```python
from build123d import *

# Parameters (mm, degrees)
SKETCH_1_R          = 9
EXTRUDE_1_DEPTH     = 8
CUT_EXTRUDE_1_DEPTH = 16.033296378
EXTRUDE_START       = -8
SKETCH_7_R          = 23
SKETCH_7_R_2        = 9
EXTRUDE_2_DEPTH     = 8
SKETCH_8_R          = 29
SKETCH_8_R_2        = 23
EXTRUDE_3_DEPTH     = 0.5
EXTRUDE_START_2     = -0.5
SKETCH_9_R          = 29
SKETCH_9_R_2        = 23
EXTRUDE_4_DEPTH     = 0.5
SKETCH_10_R         = 1.25977889
CUT_EXTRUDE_2_DEPTH = 25


with BuildPart() as part:
    # 草圖1 → 填料-伸長1 (new body)
    with BuildSketch(Plane(origin=(0, 0, 0), x_dir=(1, 0, 0), z_dir=(0, 1, 0))):
        with Locations(Location((0, 0, 0), (0, 0, 270))):
            Circle(SKETCH_1_R)
    extrude(amount=-EXTRUDE_1_DEPTH)

    # 草圖2 → 除料-伸長1 (cut, through all)
    with BuildSketch(Plane(origin=(0, -8, 0), x_dir=(-1, 0, 0), z_dir=(0, -1, 0))):
        with BuildLine():
            Line((-0.93, 1.264911064), (-0.93, -1.264911064))
            ThreePointArc((-0.93, -1.264911064), (0.708801806, -1.400892573), (1.57, 0))
            ThreePointArc((1.57, 0), (0.708801806, 1.400892573), (-0.93, 1.264911064))
        make_face()
    extrude(amount=-CUT_EXTRUDE_1_DEPTH, mode=Mode.SUBTRACT)

    # 草圖7 → 填料-伸長2 (add)
    with BuildSketch(Plane(origin=(0, -8, 0), x_dir=(-1, 0, 0), z_dir=(0, -1, 0)).offset(EXTRUDE_START)):
        with Locations(Location((0, 0, 0), (0, 0, 90))):
            Circle(SKETCH_7_R)
        Circle(SKETCH_7_R_2, mode=Mode.SUBTRACT)
    extrude(amount=EXTRUDE_2_DEPTH)

    # 草圖8 → 填料-伸長3 (add)
    with BuildSketch(Plane(origin=(0, 0, 0), x_dir=(1, 0, 0), z_dir=(0, 1, 0))):
        with Locations(Location((0, 0, 0), (0, 0, 270))):
            Circle(SKETCH_8_R)
        with Locations(Location((0, 0, 0), (0, 0, 90))):
            Circle(SKETCH_8_R_2, mode=Mode.SUBTRACT)
    extrude(amount=-EXTRUDE_3_DEPTH)

    # 草圖9 → 填料-伸長4 (add)
    with BuildSketch(Plane.XZ.offset(8).offset(EXTRUDE_START_2)):
        with Locations(Location((0, 0, 0), (0, 0, 90))):
            Circle(SKETCH_9_R)
        with Locations(Location((0, 0, 0), (0, 0, 270))):
            Circle(SKETCH_9_R_2, mode=Mode.SUBTRACT)
    extrude(amount=EXTRUDE_4_DEPTH)

    # 草圖10 → 除料-伸長2 (cut, symmetric)
    with BuildSketch(Plane(origin=(0, 0, 0), x_dir=(0, 0, -1), z_dir=(1, 0, 0))):
        with Locations((-11.0333289, -4.987601344)):
            Circle(SKETCH_10_R)
    extrude(amount=CUT_EXTRUDE_2_DEPTH, both=True, mode=Mode.SUBTRACT)


solid = part.part
```
The listing builds one solid part. Answer for the finished solid, in the listing's coordinates (mm). A direction names the side the tool comes from. Coordinates: 2 decimals unless noted, no trailing zeros. Loops run counter-clockwise (first coordinate to the right, second up) from the corner with the lowest first, then second, coordinate; pieces in that order, holes last. Notation, with made-up numbers: M 6,22.5 L 15,22.5 A14 ccw 15,33.5 Z; hole C -19.5,-25.75 d1. An arc over 180 degrees is marked long. Answer as a JSON object with one key per item and string values. Group by question number.
Item 1: Which of the six approach directions +Z, -Z, +X, -X, +Y, -Y give full straight-line access (tool end or side, diameter ignored) to faces 1 (the face through (-11.107, -0.246, 26.789)), 2 (the face through (22, -0.5, -9))?
Item 2: Section B-B (x = 10.5) is taken. Write down the section's boundary in (y, z).
Item 3: Section A-A (x = 0) is taken. Write down the section's boundary in (y, z).
Item 4: Section D-D (y = -1.25) is taken. Write down the section's boundary in (x, z).
Item 5: Section C-C (z = -8) is taken. Write down the section's boundary in (x, y), and give its area (3 significant figures).
Item 6: Each of these flat-tipped pins is pushed along its axis until it touches: P1, Ø1.3, axis at y = -5, z = 0.5, coming from the -X side; P2, Ø1.5, axis at y = -3.5, z = -22, coming from the +X side; P3, Ø2, axis at y = -4.99, z = 11.03, coming from the -X side. Where does it stop, or does it pass through?
Item 7: Determine the mould class of faces 3 (the face through (0.93, -4, 0)), 4 (the face through (-22, -7.5, -9)), 5 (the face through (0.291, -6.105, 10.452)), 6 (the face through (19.394, -3.951, -12.365)) for opening direction Z: +Z half, -Z half, draft (parallel to the pull), parting line (faces both ways), or undercut.
Item 8: Consider L1, parallel to Y at x = 23, z = 14; L2, parallel to X at y = -1, z = -16; L3, parallel to Z at x = -9, y = -1.25. Determine where each line is inside the solid, lowest interval first.
Solved:
{
 "1": {"face 1": "+Y, -Y", "face 2": "none"},
 "2": {"outline": "M -8,-27.03 L -7.5,-27.03 L -7.5,-20.46 L -0.5,-20.46 L -0.5,-27.03 L 0,-27.03 L 0,27.03 L -0.5,27.03 L -0.5,20.46 L -7.5,20.46 L -7.5,27.03 L -8,27.03 Z; hole C -4.99,11.03 d2.52"},
 "3": {"outline": "M -8,-29 L -7.5,-29 L -7.5,-23 L -0.5,-23 L -0.5,-29 L 0,-29 L 0,-1.57 L -8,-1.57 Z; M -8,1.57 L 0,1.57 L 0,29 L -0.5,29 L -0.5,23 L -7.5,23 L -7.5,29 L -8,29 Z; hole C -4.99,11.03 d2.52"},
 "4": {"outline": "C 0,0 d46; hole M 0.93,-1.26 L 0.93,1.26 A1.57 ccw long Z"},
 "5": {"outline": "M -27.87,-8 L 27.87,-8 L 27.87,-7.5 L 21.56,-7.5 L 21.56,-0.5 L 27.87,-0.5 L 27.87,0 L -27.87,0 L -27.87,-0.5 L -21.56,-0.5 L -21.56,-7.5 L -27.87,-7.5 Z", "area": "358 mm2"},
 "6": {"P1": "stops at x = -23", "P2": "stops at x = 8.8", "P3": "passes through"},
 "7": {"face 3": "undercut", "face 4": "draft", "face 5": "undercut", "face 6": "parting line"},
 "8": {"L1": "y = -8 to -7.5, -0.5 to 0", "L2": "x = -16.52 to 16.52", "L3": "z = -21.17 to 21.17"}
}
